```python
from build123d import *

# Parameters (mm, degrees)
PAD_DEPTH    = 5
POCKET_DEPTH = 5
FILLET_R     = 2.4
FILLET001_R  = 2.4


with BuildPart() as part:
    # Sketch → Pad (new body)
    with BuildSketch(Plane.XY):
        with BuildLine():
            Line((0, 0), (70, 0))
            Line((70, 0), (70, 3))
            ThreePointArc((70, 103), (49.807335, 53), (70, 3))
            Line((70, 106), (70, 103))
            Line((15, 106), (70, 106))
            Line((15, 103), (15, 106))
            Line((24, 36), (15, 103))
            Line((0, 3), (24, 36))
            Line((0, 0), (0, 3))
        make_face()
    extrude(amount=PAD_DEPTH)

    # Sketch001 → Pocket (cut)
    with BuildSketch(Plane.XY):
        Polygon((35, 96.5), (27.638784, 92.25), (27.638784, 83.75), (35, 79.5), (42.361216, 83.75), (42.361216, 92.25), align=None)
    extrude(amount=POCKET_DEPTH, mode=Mode.SUBTRACT)

    # Fillet
    fillet_edges = [part.edges().sort_by_distance(p)[0] for p in [
        (49.807335, 53, 5),
        (49.807335, 53, 0),
    ]]
    fillet(fillet_edges, radius=FILLET_R)

    # Fillet001
    fillet001_edges = [part.edges().sort_by_distance(p)[0] for p in [
        (19.5, 69.5, 5),
        (19.5, 69.5, 0),
        (12, 19.5, 5),
        (12, 19.5, 0),
    ]]
    fillet(fillet001_edges, radius=FILLET001_R)


solid = part.part
```
Part model, mm, in its own coordinate system. A direction names the side the tool comes from. Give positions to 0.01 mm unless a question says otherwise; leave off trailing zeros. Loops run counter-clockwise (first coordinate to the right, second up) from the corner with the lowest first, then second, coordinate; pieces in that order, holes last. Notation, with made-up numbers: M 54,-29 L 104,-29 A21 ccw 104,-2 Z; hole C -12,-2 d4. An arc over 180 degrees is marked long. Return JSON: item names as keys, results as strings.
1) Flat gauge pin, fed straight in: pin 1 Ø1.4 at (y, z) = (104, 2.5) entering from -X. Where does the tip first touch, or does it go through?
Calculated:
{"pin 1": "stops at x = 15"}
2) Pull direction X, two halves, no side cores. Call faces 1 (the face through (27.639, 88, 2)), 2 (the face through (42, 106, 2)), 3 (the face through (70, 1, 2)), 4 (the face through (0, 1, 2)): released by +X, released by -X, zero draft, split by the parting line, or undercut.
Calculated:
{"face 1": "undercut", "face 2": "zero draft", "face 3": "released by +X", "face 4": "released by -X"}
3) Saw through at A-A, the plane x = 30. List the corners of the cut face in (y, z), then the cut area to 3 significant figures.
Calculated:
{"outline": "M 0,0 L 82.39,0 L 82.39,5 L 0,5 Z; M 93.61,0 L 106,0 L 106,5 L 93.61,5 Z", "area": "474 mm2"}
4) Drill centre lines: line 1 (Y direction, x = 39, z = 3.8); line 2 (Y direction, x = 37.5, z = 0.4); line 3 (X direction, y = 95, z = 1.55). Where is each one in solid material? Low to high.
Calculated:
{"line 1": "y = 0 to 81.81, 94.19 to 106", "line 2": "y = 0 to 80.94, 95.06 to 106", "line 3": "x = 16.23 to 32.4, 37.6 to 63.14"}
5) 3-axis set-ups, long thin cutter, end or side, ignore diameter. For faces 5 (the face through (20, 71.1, 0.7)), 6 (the face through (38.732, 94.345, 2.465)), 7 (the face through (12.335, 18.734, 4.316)): which of +Z, -Z, +X, -X, +Y, -Y reach the whole face in a straight line?
Calculated:
{"face 5": "-Z, -X", "face 6": "+Z, -Z", "face 7": "+Z, -X"}
